Can you work these out from the model? Positions are in its coordinate system, mm. A direction names the side the tool comes from. Coordinates: 2 decimals unless noted, no trailing zeros. Loops run counter-clockwise (first coordinate to the right, second up) from the corner with the lowest first, then second, coordinate; pieces in that order, holes last.
```python
from build123d import *

# Parameters (mm, degrees)
SKETCH1_W           = 90
SKETCH1_H           = 50
BOSS_EXTRUDE1_DEPTH = 30
FILLET1_R           = 15
SKETCH2_R           = 22.703438641
BOSS_EXTRUDE2_DEPTH = 1
SKETCH3_R           = 15
CUT_EXTRUDE1_DEPTH  = 1
SKETCH4_W           = 17.5
SKETCH4_H           = 10
BOSS_EXTRUDE3_DEPTH = 1
SKETCH5_R           = 3.75
CUT_EXTRUDE2_DEPTH  = 1
SKETCH6_R           = 2.30333071
BOSS_EXTRUDE4_DEPTH = 1


with BuildPart() as part:
    # Sketch1 → Boss-Extrude1 (new body)
    with BuildSketch(Plane.XY):
        with Locations((45, 25)):
            Rectangle(SKETCH1_W, SKETCH1_H)
    extrude(amount=-BOSS_EXTRUDE1_DEPTH)

    # Fillet1
    fillet1_edges = [part.edges().sort_by_distance(p)[0] for p in [
        (0, 50, -15),
        (90, 50, -15),
        (90, 0, -15),
        (0, 0, -15),
    ]]
    fillet(fillet1_edges, radius=FILLET1_R)

    # Sketch2 → Boss-Extrude2 (add)
    with BuildSketch(Plane.XY):
        with Locations((45, 25)):
            Circle(SKETCH2_R)
    extrude(amount=BOSS_EXTRUDE2_DEPTH)

    # Sketch3 → Cut-Extrude1 (cut)
    with BuildSketch(Plane.XY.offset(1)):
        with Locations((45, 25)):
            Circle(SKETCH3_R)
    extrude(amount=-CUT_EXTRUDE1_DEPTH, mode=Mode.SUBTRACT)

    # Sketch4 → Boss-Extrude3 (add)
    with BuildSketch(Plane.XY):
        with Locations((45, 25)):
            Rectangle(SKETCH4_W, SKETCH4_H)
    extrude(amount=BOSS_EXTRUDE3_DEPTH)

    # Sketch5 → Cut-Extrude2 (cut)
    with BuildSketch(Plane.XY.offset(1)):
        with Locations((45, 25)):
            Circle(SKETCH5_R)
    extrude(amount=-CUT_EXTRUDE2_DEPTH, mode=Mode.SUBTRACT)

    # Sketch6 → Boss-Extrude4 (add)
    with BuildSketch(Plane.XY):
        with Locations((45, 25)):
            Circle(SKETCH6_R)
    extrude(amount=BOSS_EXTRUDE4_DEPTH)


solid = part.part
```
(1) I'm going to push flat-ended pins straight in: pin 1 (5 mm diameter, centred on x = 12, z = -7.5, fed in from -Y); pin 2 (1.5 mm diameter, centred on x = 66, y = 11, fed in from +Z); pin 3 (10 mm diameter, centred on y = 40.5, z = -3.5, fed in from +X). Where does each tip first touch, or does it pass through?
Check values:
pin 1: stops at y = 0.01
pin 2: stops at z = 0
pin 3: stops at x = 89.99
(2) I want a section at D-D on y = 14. Write out the boundary of the cut face in (x, z).
Check values:
outline: (0.03, -30) - (89.97, -30) - (89.97, 0) - (64.86, 0) - (64.86, 1) - (55.2, 1) - (55.2, 0) - (34.8, 0) - (34.8, 1) - (25.14, 1) - (25.14, 0) - (0.03, 0) - close
(3) I want a section at A-A on y = 25. Write out the boundary of the cut face in (x, z).
Check values:
outline: (0, -30) - (90, -30) - (90, 0) - (67.7, 0) - (67.7, 1) - (60, 1) - (60, 0) - (53.75, 0) - (53.75, 1) - (48.75, 1) - (48.75, 0) - (47.3, 0) - (47.3, 1) - (42.7, 1) - (42.7, 0) - (41.25, 0) - (41.25, 1) - (36.25, 1) - (36.25, 0) - (30, 0) - (30, 1) - (22.3, 1) - (22.3, 0) - (0, 0) - close
(4) Which directions (+Z, -Z, +X, -X, +Y, -Y) give clear straight access to the entire face, cutting with the end or side of a thin tool? Please do faces 1 (the cylindrical face through (4.28, 4.51, -15.21)), 2 (the cylindrical face through (33.1, 15.87, 0.51)).
Check values:
face 1: +Z, -Z, -X, -Y
face 2: +Z
(5) If I drill on probe 1 along Y at (x, z) = (45, 0.5); probe 2 along Z at (x, y) = (15, 6.5); probe 3 along X at (y, z) = (8, -11.5), over which ranges is the centre line in solid material (lowest first)?
Check values:
probe 1: y = 2.3 to 10, 20 to 21.25, 22.7 to 27.3, 28.75 to 30, 40 to 47.7
probe 2: z = -30 to 0
probe 3: x = 1.73 to 88.27
(6) I want a section at B-B on z = -11.5. Write out the boundary of the cut face in (x, y).
Check values:
outline: (0, 15) arc R15 ccw to (15, 0) - (75, 0) arc R15 ccw to (90, 15) - (90, 35) arc R15 ccw to (75, 50) - (15, 50) arc R15 ccw to (0, 35) - close
(7) If we mould it in two halves opening along X, with no side actions, what happens to faces 3 (the cylindrical face through (4.28, 45.49, -15.21)), 4 (the cylindrical face through (42.024, 22.718, 0.507)), 5 (the cylindrical face through (28.267, 40.344, 0.493)), 6 (the flat face through (50, 10, 1))? For each: released by +X, released by -X, zero draft, split by the parting line, or undercut.
Check values:
face 3: released by -X
face 4: undercut
face 5: split by the parting line
face 6: zero draft
(8) I want a section at C-C on x = 45. Write out the boundary of the cut face in (y, z), then the cut area to 3 significant figures.
Check values:
outline: (0, -30) - (50, -30) - (50, 0) - (47.7, 0) - (47.7, 1) - (40, 1) - (40, 0) - (30, 0) - (30, 1) - (28.75, 1) - (28.75, 0) - (27.3, 0) - (27.3, 1) - (22.7, 1) - (22.7, 0) - (21.25, 0) - (21.25, 1) - (20, 1) - (20, 0) - (10, 0) - (10, 1) - (2.3, 1) - (2.3, 0) - (0, 0) - close
area: 1,520 mm2
